Input: part model. Units: mm. Frame: model coordinates. A direction names the side the tool comes from. Coordinates: 2 decimals unless noted, no trailing zeros. Write each loop counter-clockwise with the first axis right and the second up, starting at its lowest first coordinate (ties: lowest second). Pieces come first, ordered by that corner, then holes. Notation, with made-up numbers: M 29,16.5 L 84,16.5 A13 cw 84,40.5 Z; hole C 79,21 d2. An arc over 180 degrees is marked long. Write each question's results on one line, items separated by ' | '. Start each with the question number.
1. Section query D-D, the plane z = 59. Output: boundary loops of the cut face in (x, y).
2. Pull-direction query (X, two-part tool) for faces 1 (the cylindrical face through (-13.5, 65.51, 31.43)), 2 (the cylindrical face through (62.99, -63.15, 98.6)), 3 (the cylindrical face through (-63.15, -62.99, 98.6)); classes: +X half, -X half, draft (parallel to the pull), parting line (faces both ways), or undercut.
3. First-contact query: pin 1 (0.8 mm diameter, centred on y = 65.5, z = 66, fed in from -X); pin 2 (0.5 mm diameter, centred on y = 65.5, z = 100, fed in from +X). Flat tips, straight axial feed; report the tip coordinate or a pass-through.
4. Set-up query: faces 4 (the cylindrical face through (61.99, 62.15, 98.6)), 5 (the flat face through (66, -1, 99)), 6 (the cylindrical face through (-13.57, 65.51, 128.5)). Return all of +Z, -Z, +X, -X, +Y, -Y with unobstructed straight access to the full face (end or side cutting, diameter ignored); none if empty.
5. Section query A-A, the plane y = 25. Output: boundary loops of the cut face in (x, z).
6. Section query C-C, the plane z = 14. Output: boundary loops of the cut face in (x, y), and give its area (3 significant figures).
7. Ray query, probe 1 along Z at (x, y) = (-24, 65.6); probe 2 along Y at (x, z) = (41, 34); probe 3 along Y at (x, z) = (56, 164). Return the intervals inside material, ascending.
```python
from build123d import *

# Parameters (mm, degrees)
F1_DEPTH = 200
F3_DEPTH = 25
F4_R     = 0.5
F5_DEPTH = 2


with BuildPart() as f1:
    # F0 (on Top) → F1 (new body)
    with BuildSketch(Plane.XY):
        with BuildLine():
            Line((-56, -66), (56, -66))
            ThreePointArc((56, -66), (63.071068, -63.071068), (66, -56))
            Line((66, -56), (66, 56))
            ThreePointArc((66, 56), (63.071068, 63.071068), (56, 66))
            Line((56, 66), (-56, 66))
            ThreePointArc((-56, 66), (-63.071068, 63.071068), (-66, 56))
            Line((-66, 56), (-66, -56))
            ThreePointArc((-66, -56), (-63.071068, -63.071068), (-56, -66))
        make_face()
        with BuildLine():
            Line((-55, 65), (55, 65))
            ThreePointArc((55, 65), (62.071068, 62.071068), (65, 55))
            Line((65, 55), (65, -55))
            ThreePointArc((65, -55), (62.071068, -62.071068), (55, -65))
            Line((55, -65), (-55, -65))
            ThreePointArc((-55, -65), (-62.071068, -62.071068), (-65, -55))
            Line((-65, -55), (-65, 55))
            ThreePointArc((-65, 55), (-62.071068, 62.071068), (-55, 65))
        make_face(mode=Mode.SUBTRACT)
    extrude(amount=F1_DEPTH)

    # F2 (on face) → F3 (cut)
    with BuildSketch(Plane(origin=(0, 66, 0), x_dir=(-1, 0, 0), z_dir=(0, 1, 0))):
        with BuildLine():
            Line((-10, 30), (10, 30))
            ThreePointArc((10, 30), (13.535534, 31.464466), (15, 35))
            Line((15, 35), (15, 125))
            ThreePointArc((15, 125), (13.535534, 128.535534), (10, 130))
            Line((10, 130), (-10, 130))
            ThreePointArc((-10, 130), (-13.535534, 128.535534), (-15, 125))
            Line((-15, 125), (-15, 35))
            ThreePointArc((-15, 35), (-13.535534, 31.464466), (-10, 30))
        make_face()
    extrude(amount=-F3_DEPTH, mode=Mode.SUBTRACT)

    # F4 (on face) → F5 (cut)
    with BuildSketch(Plane(origin=(0, 66, 0), x_dir=(-1, 0, 0), z_dir=(0, 1, 0))):
        with Locations((0, 2)):
            Circle(F4_R)
        with Locations((-4, 4)):
            Circle(F4_R)
        with Locations((-16, 6)):
            Circle(F4_R)
        with Locations((-8, 2)):
            Circle(F4_R)
        with Locations((-32, 6)):
            Circle(F4_R)
        with Locations((-12, 4)):
            Circle(F4_R)
        with Locations((-24, 2)):
            Circle(F4_R)
        with Locations((4, 4)):
            Circle(F4_R)
        with Locations((12, 4)):
            Circle(F4_R)
        with Locations((24, 2)):
            Circle(F4_R)
        with Locations((20, 4)):
            Circle(F4_R)
        with Locations((16, 6)):
            Circle(F4_R)
        with Locations((32, 2)):
            Circle(F4_R)
        with Locations((24, 6)):
            Circle(F4_R)
        with Locations((-16, 2)):
            Circle(F4_R)
        with Locations((-24, 6)):
            Circle(F4_R)
        with Locations((-20, 4)):
            Circle(F4_R)
        with Locations((8, 2)):
            Circle(F4_R)
        with Locations((-28, 4)):
            Circle(F4_R)
        with Locations((16, 2)):
            Circle(F4_R)
        with Locations((8, 6)):
            Circle(F4_R)
        with Locations((28, 4)):
            Circle(F4_R)
        with Locations((-8, 6)):
            Circle(F4_R)
        with Locations((0, 6)):
            Circle(F4_R)
        with Locations((32, 6)):
            Circle(F4_R)
        with Locations((-32, 2)):
            Circle(F4_R)
        with Locations((36, 4)):
            Circle(F4_R)
        with Locations((-36, 4)):
            Circle(F4_R)
    extrude(amount=-F5_DEPTH, mode=Mode.SUBTRACT)


solid = f1.part
```
Answer:
1) outline: M -66,-56 A10 ccw -56,-66 L 56,-66 A10 ccw 66,-56 L 66,56 A10 ccw 56,66 L 15,66 L 15,65 L 55,65 A10 cw 65,55 L 65,-55 A10 cw 55,-65 L -55,-65 A10 cw -65,-55 L -65,55 A10 cw -55,65 L -15,65 L -15,66 L -56,66 A10 ccw -66,56 Z
2) face 1: undercut | face 2: +X half | face 3: -X half
3) pin 1: x = -60.15 | pin 2: x = 59.8
4) face 4: +Z, -Z | face 5: +Z, -Z, +X, +Y, -Y | face 6: +Y
5) outline: M -66,0 L -65,0 L -65,200 L -66,200 Z; M 65,0 L 66,0 L 66,200 L 65,200 Z
6) outline: M -66,-56 A10 ccw -56,-66 L 56,-66 A10 ccw 66,-56 L 66,56 A10 ccw 56,66 L -56,66 A10 ccw -66,56 Z; hole M -65,-55 A10 ccw -55,-65 L 55,-65 A10 ccw 65,-55 L 65,55 A10 ccw 55,65 L -55,65 A10 ccw -65,55 Z | area: 524 mm^2
7) probe 1: 0 to 1.5, 2.5 to 5.5, 6.5 to 200 | probe 2: -66 to -65, 65 to 66 | probe 3: -66 to -64.95, 64.95 to 66
